Work out the finished part from the listing and answer in its coordinate system (mm). Face numbers are marked on the shaded views. A direction names the side the tool comes from. Coordinates: 2 decimals unless noted, no trailing zeros. Write each loop counter-clockwise with the first axis right and the second up, starting at its lowest first coordinate (ties: lowest second). Pieces come first, ordered by that corner, then holes. Notation, with made-up numbers: (54, 0) - (83, 0) arc R18 ccw to (83, 13) - close; hole circle Ø6 at (65.25, 43.5). An arc over 180 degrees is marked (long way). One line per item, written item: value.
Autodesk Inventor part; units mm, degrees
ref_plane "YZ Plane" through (0, 0, 0) normal (1, 0, 0) x (0, 1, 0)
ref_plane "XZ Plane" through (0, 0, 0) normal (0, 1, 0) x (-1, 0, 0)
ref_plane "XY Plane" through (0, 0, 0) normal (0, 0, 1) x (1, 0, 0)
ref_plane "Work Plane1" through (0, 0, 0) normal (0, 0, 1) x (1, 0, 0)
sketch "Sketch1" plane through (0, 0, 0) normal (0, 0, 1) x (1, 0, 0)
  line L0 (45, 75) -> (-45, 75)
  line L1 (-50, 70) -> (-50, -70)
  line L2 (-45, -75) -> (45, -75)
  line L3 (50, -70) -> (50, 70)
  arc A0 (50, 70) -> (45, 75) centre (45, 70) ccw
  arc A1 (-45, 75) -> (-50, 70) centre (-45, 70) ccw
  arc A2 (-50, -70) -> (-45, -75) centre (-45, -70) ccw
  arc A3 (45, -75) -> (50, -70) centre (45, -70) ccw
  line L4 (43.008, 67.9028) -> (-43.1443, 67.9028)
  line L5 (-43.1443, 67.9028) -> (-43.1443, -67.7709)
  line L6 (-43.1443, -67.7709) -> (43.008, -67.7709)
  line L7 (43.008, -67.7709) -> (43.008, 67.9028)
  circle A4 centre (45, 70) radius 1.5085
  circle A5 centre (-45, 70) radius 1.5
  circle A6 centre (-45, -70) radius 1.5
  circle A7 centre (45, -70) radius 1.5
  point P0 (0, 0)
  dimension "d0" = 5
  dimension "d1" = 3
  dimension "d2" = 3
  dimension "d3" = 3
extrude "Extrusion1" add sketch "Sketch1" along normal blind 60
sketch "Sketch2" plane through (50, -70, 0) normal (1, 0, 0) x (0, 0, -1)
  circle A0 centre (-27.4102, 19.5745) radius 12.5
  circle A1 centre (-27.4102, 112.7876) radius 3.75
  point P0 (0, 70)
  dimension "d6" = 25
  dimension "d9" = 7.5
extrude "Extrusion2" cut sketch "Sketch2" against normal up to surface (6.992 mm away)
sketch "Sketch3" plane through (0, 0, 60) normal (0, 0, 1) x (1, 0, 0)
  line L0 (-45, 75) -> (45, 75)
  line L1 (50, 70) -> (50, -70)
  line L2 (45, -75) -> (-45, -75)
  line L3 (-50, -70) -> (-50, 70)
  arc A0 (45, -75) -> (50, -70) centre (45, -70) ccw
  arc A1 (-50, -70) -> (-45, -75) centre (-45, -70) ccw
  arc A2 (-45, 75) -> (-50, 70) centre (-45, 70) ccw
  arc A3 (50, 70) -> (45, 75) centre (45, 70) ccw
  point P0 (0, 0)
  dimension "d10" = 5
extrude "Extrusion3" add sketch "Sketch3" along normal blind 3.5625
sketch "Sketch4" plane through (-50, -70, 0) normal (-1, 0, 0) x (0, 0, 1)
  circle A0 centre (33.4987, 16.7277) radius 5.1927
  circle A1 centre (33.4987, 109.0376) radius 6.5
  point P0 (0, 70)
  dimension "d15" = 13
extrude "Extrusion4" cut sketch "Sketch4" against normal up to surface (6.8557 mm away)
properties part number "Base"
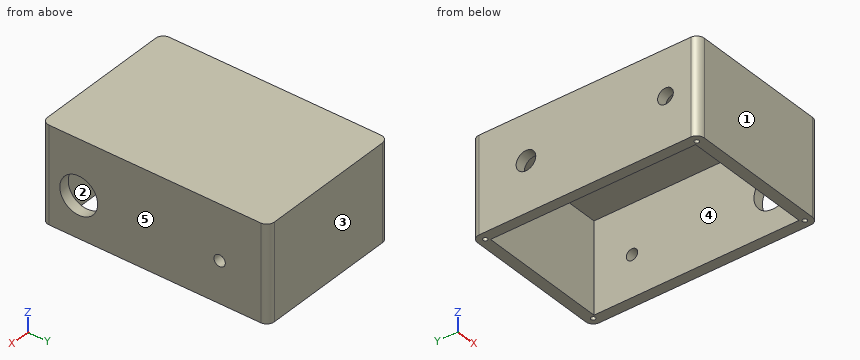
Item 1: Section C-C, the plane x = -36 is taken. Determine the outline of the cut face in (y, z), then the cut area to 3 significant figures.
Evaluation:
outline: (-75, 0) - (-67.77, 0) - (-67.77, 60) - (67.9, 60) - (67.9, 0) - (75, 0) - (75, 63.56) - (-75, 63.56) - close
area: 1,390 mm2
Item 2: Given pin 1 (2.5 mm diameter, centred on x = -45, y = 70, fed in from -Z), flat-ended and moving along its own axis, determine where the tip first touches the part or whether it passes through.
Evaluation:
pin 1: stops at z = 60
Item 3: Section A-A, the plane z = 52 is taken. Determine the outline of the cut face in (x, y), then the cut area to 3 significant figures.
Evaluation:
outline: (-50, -70) arc R5 ccw to (-45, -75) - (45, -75) arc R5 ccw to (50, -70) - (50, 70) arc R5 ccw to (45, 75) - (-45, 75) arc R5 ccw to (-50, 70) - close; hole circle Ø3 at (-45, -70); hole circle Ø3 at (-45, 70); hole (-43.14, -67.77) - (43.01, -67.77) - (43.01, 67.9) - (-43.14, 67.9) - close; hole circle Ø3.02 at (45, 70); hole circle Ø3 at (45, -70)
area: 3,260 mm2
Item 4: Section D-D, the plane y = 8.5 is taken. Determine the outline of the cut face in (x, z), then the cut area to 3 significant figures.
Evaluation:
outline: (-50, 0) - (-43.14, 0) - (-43.14, 60) - (43.01, 60) - (43.01, 0) - (50, 0) - (50, 63.56) - (-50, 63.56) - close
area: 1,190 mm2
Item 5: Determine the mould class of the marked faces 3, 4 and 5 for opening direction X: +X half, -X half, draft (parallel to the pull), parting line (faces both ways), or undercut.
Evaluation:
face 3: draft
face 4: undercut
face 5: +X half
Item 6: Section B-B, the plane y = -44 is taken. Determine the outline of the cut face in (x, z), then the cut area to 3 significant figures.
Evaluation:
outline: (-50, 0) - (-43.14, 0) - (-43.14, 60) - (43.01, 60) - (43.01, 38.13) - (50, 38.13) - (50, 63.56) - (-50, 63.56) - close; (43.01, 0) - (50, 0) - (50, 16.69) - (43.01, 16.69) - close
area: 1,040 mm2
Item 7: Consider probe 1 along X at (y, z) = (70, 30); probe 2 along X at (y, z) = (-27, 5); probe 3 along Y at (x, z) = (-44, 49.5). Determine where each line is inside the solid, lowest interval first.
Evaluation:
probe 1: x = -50 to -46.5, -43.5 to 43.49, 46.51 to 50
probe 2: x = -50 to -43.14, 43.01 to 50
probe 3: y = -75 to -71.12, -68.88 to 68.88, 71.12 to 75
Item 8: Which of the six approach directions +Z, -Z, +X, -X, +Y, -Y give full straight-line access (tool end or side, diameter ignored) to the marked faces 1 and 2?
Evaluation:
face 1: +Z, -Z, +X, -X, -Y
face 2: -Z
